from build123d import *

# Parameters (mm, degrees)
PAD_DEPTH    = 15
POCKET_DEPTH = 8
PAD001_DEPTH = 15


with BuildPart() as part:
    # Sketch → Pad (new body)
    with BuildSketch(Plane.XY):
        with BuildLine():
            Line((-50.61699, -37.307126), (11.75, -37.307126))
            ThreePointArc((11.75, -37.307126), (12.81066, -36.867787), (13.25, -35.807126))
            Line((13.25, -35.807126), (13.25, 26.297858))
            ThreePointArc((13.25, 26.297858), (13.026109, 27.08624), (12.421272, 27.639273))
            Line((12.421272, 27.639273), (-9.578728, 38.648541))
            ThreePointArc((-9.578728, 38.648541), (-11.038382, 38.583235), (-11.75, 37.307126))
            Line((-11.75, 37.307126), (-11.75, -12.307126))
            Line((-11.75, -12.307126), (-61.073474, -12.307126))
            ThreePointArc((-61.073474, -12.307126), (-62.341517, -13.005836), (-62.428236, -14.451037))
            Line((-62.428236, -14.451037), (-51.971751, -36.451037))
            ThreePointArc((-51.971751, -36.451037), (-51.418281, -37.075169), (-50.61699, -37.307126))
        make_face()
    extrude(amount=PAD_DEPTH)

    # Sketch001 (on DatumPlane) → Pocket (cut)
    with BuildSketch(Plane.XY.offset(11.5)):
        Polygon((-8.25, -15.807126), (-57.928236, -15.807126), (-49.971751, -33.807126), (9.75, -33.807126), (9.75, 25.639273), (-8.25, 34.148541), align=None)
    extrude(amount=-POCKET_DEPTH, mode=Mode.SUBTRACT)

    # Sketch002 (on Face5 of Pocket) → Pad001 (join)
    with BuildSketch(Plane.XY.offset(15)):
        Polygon((-33.723206, -37.307126), (-28.723206, -37.307126), (13.25, 4.692874), (13.25, 9.692874), align=None)
    extrude(amount=-PAD001_DEPTH)


solid = part.part
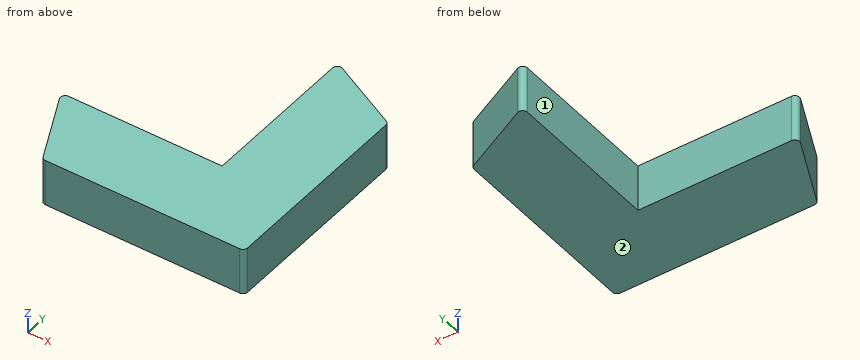
The model under review builds one solid part; all positions refer to its coordinate system, in mm. Face numbers are marked on the shaded views. A direction names the side the tool comes from. Round coordinates to 2 decimals unless told otherwise and drop trailing zeros. Loops run counter-clockwise (first coordinate to the right, second up) from the corner with the lowest first, then second, coordinate; pieces in that order, holes last. Notation, with made-up numbers: (78, 78) -> (103, 78) arc R16 ccw to (103, 109) -> close; hole circle Ø11 at (31.25, 80.5). An arc over 180 degrees is marked (long way). One line per question, with ' | ' between items. Start each with the question number.
Item 1: Wall thickness on line 1 along Y through (x, z) = (3.5, 8); line 2 along Z through (x, y) = (5.5, 23.5); line 3 along Y through (x, z) = (7, 4.5): over which ranges is each line inside the solid? List them lowest first. Write a range as [from, to].
Item 2: Add section D-D, the plane z = 8.75. Write out the cut boundary in (x, y).
Item 3: Add section A-A, the plane z = 13.75. Write out the cut boundary in (x, y), then the cut area to 3 significant figures.
Item 4: Machinability: for the marked faces 1 and 2, which of the approach directions +Z, -Z, +X, -X, +Y, -Y give a long, thin tool a straight path to every point of the face, cutting with its end or side? Answer none if there is none.
Item 5: For pin 1 (4 mm diameter, centred on x = -14, z = 8.5, fed in from +Y); pin 2 (7.5 mm diameter, centred on y = 21.5, z = 8.5, fed in from -X); pin 3 (9 mm diameter, centred on y = -22.5, z = 6, fed in from -X), all flat-tipped, find the tip position at first contact; note any pin that passes through.
Item 6: Add section B-B, the plane y = 20.5. Write out the cut boundary in (x, z).
Item 7: Add section C-C, the plane x = -31.5. Write out the cut boundary in (y, z), then the cut area to 3 significant figures.
Return value:
1) line 1: y = [-37.31, -33.81], [-5.06, -0.06], [28.59, 32.1] | line 2: z = [0, 3.5], [11.5, 15] | line 3: y = [-37.31, -33.81], [-1.56, 3.44], [26.94, 30.35]
2) outline: (-62.43, -14.45) -> (-51.97, -36.45) arc R1.5 ccw to (-50.62, -37.31) -> (11.75, -37.31) arc R1.5 ccw to (13.25, -35.81) -> (13.25, 26.3) arc R1.5 ccw to (12.42, 27.64) -> (-9.58, 38.65) arc R1.5 ccw to (-11.75, 37.31) -> (-11.75, -12.31) -> (-61.07, -12.31) arc R1.5 ccw to start; hole (-57.93, -15.81) -> (-49.97, -33.81) -> (-30.23, -33.81) -> (-12.24, -15.81) -> close; hole (-25.23, -33.81) -> (9.75, -33.81) -> (9.75, 1.19) -> close; hole (-8.25, -11.82) -> (9.75, 6.19) -> (9.75, 25.64) -> (-8.25, 34.15) -> close
3) outline: (-62.43, -14.45) -> (-51.97, -36.45) arc R1.5 ccw to (-50.62, -37.31) -> (11.75, -37.31) arc R1.5 ccw to (13.25, -35.81) -> (13.25, 26.3) arc R1.5 ccw to (12.42, 27.64) -> (-9.58, 38.65) arc R1.5 ccw to (-11.75, 37.31) -> (-11.75, -12.31) -> (-61.07, -12.31) arc R1.5 ccw to start | area: 2,910 mm2
4) face 1: +Z, -Z, -X, +Y | face 2: -Z, +X, -X, +Y, -Y
5) pin 1: stops at y = -12.31 | pin 2: stops at x = -11.75 | pin 3: stops at x = -60.74
6) outline: (-11.75, 0) -> (13.25, 0) -> (13.25, 15) -> (-11.75, 15) -> close; hole (-8.25, 3.5) -> (9.75, 3.5) -> (9.75, 11.5) -> (-8.25, 11.5) -> close
7) outline: (-37.31, 0) -> (-12.31, 0) -> (-12.31, 15) -> (-37.31, 15) -> close; hole (-33.81, 3.5) -> (-15.81, 3.5) -> (-15.81, 11.5) -> (-33.81, 11.5) -> close | area: 231 mm2
